from build123d import *

# Parameters (mm, degrees)
SKETCH_1_W          = 103
SKETCH_1_H          = 90.5
EXTRUDE_1_DEPTH     = 6.5
SKETCH_2_W          = 9
SKETCH_2_H          = 14
SKETCH_2_W_2        = 16
SKETCH_2_H_2        = 14.5
SKETCH_2_W_3        = 13
SKETCH_2_H_3        = 17.5
SKETCH_2_H_4        = 21
SKETCH_2_H_5        = 10
SKETCH_2_W_4        = 69.5
SKETCH_2_H_6        = 50
SKETCH_2_R          = 18
SKETCH_2_W_5        = 2.5
SKETCH_2_H_7        = 19
SKETCH_2_W_6        = 5
SKETCH_2_H_8        = 50.5
EXTRUDE_2_DEPTH     = 27.5
CUT_EXTRUDE_1_REACH = 143.263
SKETCH_3_W          = 9
SKETCH_3_H          = 16.5
SKETCH_3_W_2        = 16
SKETCH_3_H_2        = 21
SKETCH_3_W_3        = 13
SKETCH_3_H_3        = 10.5
SKETCH_3_H_4        = 14
SKETCH_3_H_5        = 24.5
SKETCH_4_W          = 69.5
SKETCH_4_H          = 9
CUT_EXTRUDE_2_DEPTH = 17.5
SKETCH_5_R          = 1.55
CUT_EXTRUDE_3_DEPTH = 140.840981118
CUT_EXTRUDE_4_REACH = 135.8
SKETCH_6_W          = 21
SKETCH_6_H          = 19
CUT_EXTRUDE_5_REACH = 141.091
SKETCH_7_W          = 16
SKETCH_7_H          = 50.5
FILLET_1_R          = 2


with BuildPart() as part:
    # 草图1 → 凸台-拉伸1 (new body)
    with BuildSketch(Plane.XY):
        with Locations((51.5, 45.25)):
            Rectangle(SKETCH_1_W, SKETCH_1_H)
    extrude(amount=EXTRUDE_1_DEPTH)

    # 草图2 → 凸台-拉伸2 (add)
    # profile 1 of 9: a face of its own
    with BuildSketch(Plane.XY.offset(6.5)):
        with Locations((7.5, 7)):
            Rectangle(SKETCH_2_W, SKETCH_2_H)
    # profile 2 of 9: a face of its own
    with BuildSketch(Plane.XY.offset(6.5)):
        with Locations((24, 7.25)):
            Rectangle(SKETCH_2_W_2, SKETCH_2_H_2)
    # profile 3 of 9: a face of its own
    with BuildSketch(Plane.XY.offset(6.5)):
        with Locations((42.5, 8.75)):
            Rectangle(SKETCH_2_W_3, SKETCH_2_H_3)
    # profile 4 of 9: a face of its own
    with BuildSketch(Plane.XY.offset(6.5)):
        with Locations((59.5, 8.75)):
            Rectangle(SKETCH_2_W_3, SKETCH_2_H_3)
    # profile 5 of 9: a face of its own
    with BuildSketch(Plane.XY.offset(6.5)):
        with Locations((77, 10.5)):
            Rectangle(SKETCH_2_W_2, SKETCH_2_H_4)
    # profile 6 of 9: a face of its own
    with BuildSketch(Plane.XY.offset(6.5)):
        with Locations((93.5, 5)):
            Rectangle(SKETCH_2_W, SKETCH_2_H_5)
    # profile 7 of 9: a face of its own
    with BuildSketch(Plane.XY.offset(6.5)):
        with Locations((48.75, 55.5)):
            Rectangle(SKETCH_2_W_4, SKETCH_2_H_6)
        with Locations((48.75, 60)):
            Circle(SKETCH_2_R, mode=Mode.SUBTRACT)
    # profile 8 of 9: a face of its own
    with BuildSketch(Plane.XY.offset(6.5)):
        with Locations((91.25, 58)):
            Rectangle(SKETCH_2_W_5, SKETCH_2_H_7)
    # profile 9 of 9: a face of its own
    with BuildSketch(Plane.XY.offset(6.5)):
        with Locations((97.5, 47.25)):
            Rectangle(SKETCH_2_W_6, SKETCH_2_H_8)
    extrude(amount=EXTRUDE_2_DEPTH)

    # 草图3 → 切除-拉伸1 (cut, up to next)
    with BuildSketch(Plane.XZ, mode=Mode.PRIVATE) as cut_extrude_1_sk1:
        with Locations((7.5, 25.75)):
            Rectangle(SKETCH_3_W, SKETCH_3_H)
    cut_extrude_1_tool1 = extrude(cut_extrude_1_sk1.sketch, amount=-CUT_EXTRUDE_1_REACH, mode=Mode.PRIVATE) & part.part
    # 草图3 → 切除-拉伸1 (cut, up to next)
    with BuildSketch(Plane.XZ, mode=Mode.PRIVATE) as cut_extrude_1_sk2:
        with Locations((24, 23.5)):
            Rectangle(SKETCH_3_W_2, SKETCH_3_H_2)
    cut_extrude_1_tool2 = extrude(cut_extrude_1_sk2.sketch, amount=-CUT_EXTRUDE_1_REACH, mode=Mode.PRIVATE) & part.part
    # 草图3 → 切除-拉伸1 (cut, up to next)
    with BuildSketch(Plane.XZ, mode=Mode.PRIVATE) as cut_extrude_1_sk3:
        with Locations((42.5, 28.75)):
            Rectangle(SKETCH_3_W_3, SKETCH_3_H_3)
    cut_extrude_1_tool3 = extrude(cut_extrude_1_sk3.sketch, amount=-CUT_EXTRUDE_1_REACH, mode=Mode.PRIVATE) & part.part
    # 草图3 → 切除-拉伸1 (cut, up to next)
    with BuildSketch(Plane.XZ, mode=Mode.PRIVATE) as cut_extrude_1_sk4:
        with Locations((59.5, 28.75)):
            Rectangle(SKETCH_3_W_3, SKETCH_3_H_3)
    cut_extrude_1_tool4 = extrude(cut_extrude_1_sk4.sketch, amount=-CUT_EXTRUDE_1_REACH, mode=Mode.PRIVATE) & part.part
    # 草图3 → 切除-拉伸1 (cut, up to next)
    with BuildSketch(Plane.XZ, mode=Mode.PRIVATE) as cut_extrude_1_sk5:
        with Locations((77, 27)):
            Rectangle(SKETCH_3_W_2, SKETCH_3_H_4)
    cut_extrude_1_tool5 = extrude(cut_extrude_1_sk5.sketch, amount=-CUT_EXTRUDE_1_REACH, mode=Mode.PRIVATE) & part.part
    # 草图3 → 切除-拉伸1 (cut, up to next)
    with BuildSketch(Plane.XZ, mode=Mode.PRIVATE) as cut_extrude_1_sk6:
        with Locations((93.5, 21.75)):
            Rectangle(SKETCH_3_W, SKETCH_3_H_5)
    cut_extrude_1_tool6 = extrude(cut_extrude_1_sk6.sketch, amount=-CUT_EXTRUDE_1_REACH, mode=Mode.PRIVATE) & part.part
    add(cut_extrude_1_tool1.solids().sort_by_distance((7.5, 0, 25.75))[0], mode=Mode.SUBTRACT)
    add(cut_extrude_1_tool2.solids().sort_by_distance((24, 0, 23.5))[0], mode=Mode.SUBTRACT)
    add(cut_extrude_1_tool3.solids().sort_by_distance((42.5, 0, 28.75))[0], mode=Mode.SUBTRACT)
    add(cut_extrude_1_tool4.solids().sort_by_distance((59.5, 0, 28.75))[0], mode=Mode.SUBTRACT)
    add(cut_extrude_1_tool5.solids().sort_by_distance((77, 0, 27))[0], mode=Mode.SUBTRACT)
    add(cut_extrude_1_tool6.solids().sort_by_distance((93.5, 0, 21.75))[0], mode=Mode.SUBTRACT)

    # 草图4 → 切除-拉伸2 (cut)
    with BuildSketch(Plane.XY.offset(34)):
        with Locations((48.75, 35)):
            Rectangle(SKETCH_4_W, SKETCH_4_H)
    extrude(amount=-CUT_EXTRUDE_2_DEPTH, mode=Mode.SUBTRACT)

    # 草图5 → 切除-拉伸3 (cut, through all)
    with BuildSketch(Plane.XY.offset(6.5)):
        with Locations((92, 19)):
            Circle(SKETCH_5_R)
        with Locations((92, 76.5)):
            Circle(SKETCH_5_R)
        with Locations((6.5, 76.5)):
            Circle(SKETCH_5_R)
        with Locations((6.5, 19.5)):
            Circle(SKETCH_5_R)
    extrude(amount=-CUT_EXTRUDE_3_DEPTH, mode=Mode.SUBTRACT)

    # 草图6 → 切除-拉伸4 (cut, up to next)
    with BuildSketch(Plane(origin=(92.5, 0, 0), x_dir=(0, 0, -1), z_dir=(1, 0, 0)), mode=Mode.PRIVATE) as cut_extrude_4_sk1:
        with Locations((-23.5, 58)):
            Rectangle(SKETCH_6_W, SKETCH_6_H)
    cut_extrude_4_tool1 = extrude(cut_extrude_4_sk1.sketch, amount=-CUT_EXTRUDE_4_REACH, mode=Mode.PRIVATE) & part.part
    add(cut_extrude_4_tool1.solids().sort_by_distance((92.5, 58, 23.5))[0], mode=Mode.SUBTRACT)

    # 草图7 → 切除-拉伸5 (cut, up to next)
    with BuildSketch(Plane(origin=(100, 0, 0), x_dir=(0, 0, -1), z_dir=(1, 0, 0)), mode=Mode.PRIVATE) as cut_extrude_5_sk1:
        with Locations((-26, 47.25)):
            Rectangle(SKETCH_7_W, SKETCH_7_H)
    cut_extrude_5_tool1 = extrude(cut_extrude_5_sk1.sketch, amount=-CUT_EXTRUDE_5_REACH, mode=Mode.PRIVATE) & part.part
    add(cut_extrude_5_tool1.solids().sort_by_distance((100, 47.25, 26))[0], mode=Mode.SUBTRACT)

    # 圆角1
    fillet_1_edges = [part.edges().sort_by_distance(p)[0] for p in [
        (0, 90.5, 3.25),
        (103, 90.5, 3.25),
        (103, 0, 3.25),
        (0, 0, 3.25),
    ]]
    fillet(fillet_1_edges, radius=FILLET_1_R)


solid = part.part
Verification items for the finished model (mm, model axes). A direction names the side the tool comes from. Round coordinates to 2 decimals unless told otherwise and drop trailing zeros. Order: outer loops, then holes, each group sorted by start corner. A loop starts at its lowest first (then second) coordinate and runs counter-clockwise, first axis right, second up.
1. Section check C-C on x = 22. Record the cut outline in (y, z).
Final values:
outline: (0, 0) - (90.5, 0) - (90.5, 6.5) - (80.5, 6.5) - (80.5, 34) - (39.5, 34) - (39.5, 16.5) - (30.5, 16.5) - (30.5, 6.5) - (14.5, 6.5) - (14.5, 13) - (0, 13) - close
2. Thickness scan on L1, parallel to Y at x = 6.5, z = 3.25; L2, parallel to Y at x = 92, z = 3.25; L3, parallel to X at y = 45, z = 14.5. Record the ranges inside material, lowest first.
Final values:
L1: y = 0 to 17.95, 21.05 to 74.95, 78.05 to 90.5
L2: y = 0 to 17.45, 20.55 to 74.95, 78.05 to 90.5
L3: x = 14 to 38.8, 58.7 to 83.5, 95 to 100
3. Section check A-A on z = 11.5. State how many separate pieces and enclosed holes the cut face has, then the cut area to 3 significant figures.
Final values:
separate pieces: 8
enclosed holes: 1
area: 3,910 mm2
4. Section check D-D on y = 76.5. Record the cut outline in (x, z), then the cut area to 3 significant figures.
Final values:
outline: (0, 0) - (4.95, 0) - (4.95, 6.5) - (0, 6.5) - close; (8.05, 0) - (90.45, 0) - (90.45, 6.5) - (83.5, 6.5) - (83.5, 34) - (55.94, 34) - (55.94, 6.5) - (41.56, 6.5) - (41.56, 34) - (14, 34) - (14, 6.5) - (8.05, 6.5) - close; (93.55, 0) - (103, 0) - (103, 6.5) - (93.55, 6.5) - close
area: 2,140 mm2
5. Release check for a two-part mould opening along X. For faces 4 (the flat face through (3, 7, 12)), 5 (the flat face through (100, 47, 12)), 6 (the flat face through (77, 10, 20)), 7 (the flat face through (16, 7, 10)) record: +X half, -X half, draft (parallel to the pull), parting line (faces both ways), or undercut.
Final values:
face 4: -X half
face 5: +X half
face 6: draft
face 7: undercut
6. Go/stop test with flat-tipped pins: P1, Ø14.5, axis at x = 56.5, y = 8, coming from the +Z side; P2, Ø8, axis at x = 71, z = 20.5, coming from the +Y side; P3, Ø5.5, axis at y = 10, z = 14, coming from the +X side. Record where each tip stops, or that it passes through.
Final values:
P1: stops at z = 23.5
P2: stops at y = 80.5
P3: stops at x = 85
7. Access from +Z, -Z, +X, -X, +Y, -Y to the whole of each face (thin tool, end or side, straight path). Record for faces 1 (the flat face through (97, 22, 12)), 2 (the flat face through (92.5, 58, 10)), 3 (the flat face through (24, 14.5, 10)).
Final values:
face 1: +Z, +X, -X
face 2: +Z, +Y
face 3: +Z, -X
8. Section check B-B on y = 60. Record the cut outline in (x, z), then the cut area to 3 significant figures.
Final values:
outline: (0, 0) - (103, 0) - (103, 6.5) - (100, 6.5) - (100, 18) - (95, 18) - (95, 6.5) - (92.5, 6.5) - (92.5, 13) - (90, 13) - (90, 6.5) - (83.5, 6.5) - (83.5, 34) - (66.75, 34) - (66.75, 6.5) - (30.75, 6.5) - (30.75, 34) - (14, 34) - (14, 6.5) - (0, 6.5) - close
area: 1,660 mm2
